from build123d import *

# Parameters (mm, degrees)
SKETCH011_R          = 10.625
SKETCH011_R_2        = 10.25
PAD003_DEPTH         = 200
SKETCH018_R          = 4
POCKET008_DEPTH      = 50
POCKET008_DEPTH_BACK = 50
POCKET009_DEPTH      = 3


with BuildPart() as part:
    # Sketch011 → Pad003 (new body)
    with BuildSketch(Plane.XZ):
        Circle(SKETCH011_R)
        Circle(SKETCH011_R_2, mode=Mode.SUBTRACT)
    extrude(amount=PAD003_DEPTH)

    # Sketch018 → Pocket008 (cut, two sides)
    with BuildSketch(Plane.XY) as pocket008_sk:
        with Locations((0, -15.434778)):
            Circle(SKETCH018_R)
    extrude(amount=-POCKET008_DEPTH, mode=Mode.SUBTRACT)
    extrude(pocket008_sk.sketch, amount=POCKET008_DEPTH_BACK, mode=Mode.SUBTRACT)

    # Sketch019 → Pocket009 (cut)
    with BuildSketch(Plane.XZ):
        Polygon((12, -2), (12, 2), (2, 2), (2, 12), (-2, 12), (-2, 2), (-12, 2), (-12, -2), (-2, -2), (-2, -12), (2, -12), (2, -2), align=None)
    extrude(amount=POCKET009_DEPTH, mode=Mode.SUBTRACT)


with BuildPart() as part_1:
    # Body003 placement: moved
    add(part.part.moved(Location((0, 2.5, 0))))


solid = part_1.part
The model under review builds one solid part; all positions refer to its coordinate system, in mm. Coordinates: 2 decimals unless noted, no trailing zeros. Write each loop counter-clockwise with the first axis right and the second up, starting at its lowest first coordinate (ties: lowest second). Pieces come first, ordered by that corner, then holes. Notation, with made-up numbers: (50.5, 66.25) - (68.5, 66.25) arc R15 cw to (68.5, 85.25) - close; hole circle Ø8 at (-38.5, -23.5). An arc over 180 degrees is marked (long way). Answer as CSV lines item,"result".
(1) Clearance check with flat-ended pins moving along their axes: pin 1 Ø1 at (x, y) = (-7, -63) entering from -Z; pin 2 Ø0.5 at (x, z) = (-0.5, 10.5) entering from +Y; pin 3 Ø3 at (y, z) = (-41.5, -7.5) entering from +X. State where each tip first meets the part, or that it passes through.
Data:
pin 1,"stops at z = -8.4"
pin 2,"stops at y = -0.5"
pin 3,"stops at x = 8.77"
(2) We need section A-A (x = 0). Give the boundary of the cut face in (y, z) (3 decimals), plus the area to 3 significant figures.
Data:
outline,"(-197.5, -10.625) - (-16.935, -10.625) - (-16.935, -10.25) - (-197.5, -10.25) - close; (-197.5, 10.25) - (-16.935, 10.25) - (-16.935, 10.625) - (-197.5, 10.625) - close; (-8.935, -10.625) - (-0.5, -10.625) - (-0.5, -10.25) - (-8.935, -10.25) - close; (-8.935, 10.25) - (-0.5, 10.25) - (-0.5, 10.625) - (-8.935, 10.625) - close"
area,"142 mm2"
(3) We need section B-B (z = 0). Give the boundary of the cut face in (x, y) (3 decimals).
Data:
outline,"(-10.625, -197.5) - (-10.25, -197.5) - (-10.25, -0.5) - (-10.625, -0.5) - close; (10.25, -197.5) - (10.625, -197.5) - (10.625, -0.5) - (10.25, -0.5) - close"
(4) For line 1 along Y through (x, z) = (0, 10.3); line 2 along X through (y, z) = (-152, 0) (3 decimals), list the stretches that pass through material, from the lowest coordinate up. Write a range as [from, to].
Data:
line 1,"y = [-197.5, -16.93], [-8.93, -0.5]"
line 2,"x = [-10.625, -10.25], [10.25, 10.625]"
(5) We need section D-D (z = -7.5). Give the boundary of the cut face in (x, y).
Data:
outline,"(-7.53, -197.5) - (-6.99, -197.5) - (-6.99, 2.5) - (-7.53, 2.5) - close; (6.99, -197.5) - (7.53, -197.5) - (7.53, 2.5) - (6.99, 2.5) - close"
(6) We need section C-C (y = -105.5). Give the boundary of the cut face in (x, z) (3 decimals).
Data:
outline,"circle Ø21.25 at (0, 0); hole circle Ø20.5 at (0, 0)"
(7) Mouldability with a two-part tool opening along Z and no side actions: class faces 1 (the cylindrical face through (-8.43, -96.1, -6.47)), 2 (the cylindrical face through (-2.222, -96.1, -10.006)), 3 (the flat face through (7.4, 2.5, -7.4)) as pulls with the +Z half, pulls with the -Z half, needs draft (parallel to the pull), parting line crosses it, or undercut.
Data:
face 1,"parting line crosses it"
face 2,"undercut"
face 3,"needs draft"
